Autodesk Inventor part; units mm, degrees
ref_plane "YZ Plane" through (0, 0, 0) normal (1, 0, 0) x (0, 1, 0)
ref_plane "XZ Plane" through (0, 0, 0) normal (0, 1, 0) x (-1, 0, 0)
ref_plane "XY Plane" through (0, 0, 0) normal (0, 0, 1) x (1, 0, 0)
sketch "Sketch1" plane through (0, 0, 0) normal (0, 0, 1) x (1, 0, 0)
  line L0 (0, 2.4078) -> (0, -18.8352)
  line L1 (-12.7, 4.1621) -> (-12.7, -19.6361)
  line L2 (-20.3324, 0) -> (-11.9249, 0)
  circle A0 centre (-12.7, 12.7) radius 3.175
  circle A1 centre (-12.7, -12.7) radius 3.175
  line L3 (-26.1938, 25.4) -> (-0.7938, 25.4)
  line L4 (-0.7938, 25.4) -> (-0.7937, -25.4)
  line L5 (-0.7937, -25.4) -> (-26.1937, -25.4)
  line L6 (-26.1937, -25.4) -> (-26.1938, 25.4)
  point P0 (0, 0)
  dimension "d0" = 12.7
  dimension "d1" = 25.4
  dimension "d2" = 25.4
  dimension "d3" = 6.35
  dimension "d4" = 6.35
  dimension "d5" = 1.5875
  dimension "d6" = 25.4
  dimension "d7" = 50.8
  dimension "d8" = 12.7
extrude "Extrusion1" add sketch "Sketch1" along normal blind 6.35
sketch "Sketch2" plane through (0, 0, 6.35) normal (0, 0, 1) x (1, 0, 0)
  line L0 (-0.7938, 25.4) -> (-26.1938, 25.4)
  line L1 (-0.7937, -25.4) -> (-0.7938, 25.4)
  line L2 (-5.8738, 25.4) -> (-0.7937, 25.4)
  line L3 (-0.7937, 25.4) -> (-0.7937, -25.4)
  line L4 (-0.7937, -25.4) -> (-5.8737, -25.4)
  line L5 (-5.8737, -25.4) -> (-5.8738, 25.4)
  point P0 (0, 0)
  dimension "d11" = 5.08
extrude "Extrusion2" add sketch "Sketch2" along normal blind 12.7
properties part number "diffuser holder"
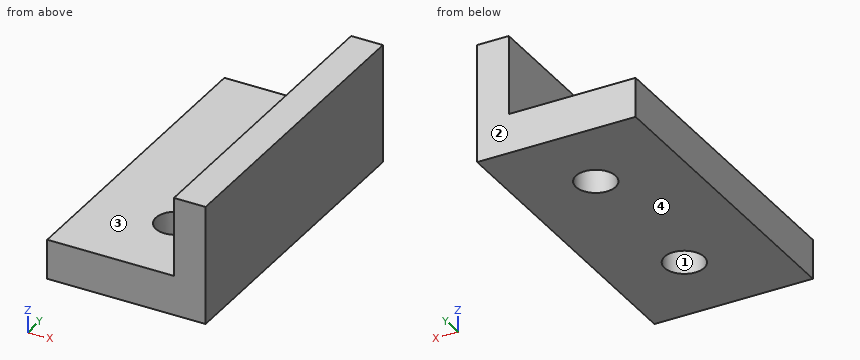
Here's how the part is built. I have some questions about the finished solid (model axes, mm). Face numbers are marked on the shaded views. A direction names the side the tool comes from. Round coordinates to 2 decimals unless told otherwise and drop trailing zeros. Write each loop counter-clockwise with the first axis right and the second up, starting at its lowest first coordinate (ties: lowest second). Pieces come first, ordered by that corner, then holes.
1. Suppose I cut it at A-A (x = -12.7). List the corners of the cut face in (y, z) for me (3 decimals), and give its area (3 significant figures).
2. Will these pins go through, and if not, where does the flat tip stop? pin 1 Ø12 at (x, y) = (-14, -10) entering from +Z; pin 2 Ø10 at (x, y) = (-20.5, -11) entering from -Z; pin 3 Ø6.5 at (y, z) = (-12.5, 15.5) entering from -X; pin 4 Ø5 at (x, y) = (-12.7, -12.7) entering from -Z.
3. I need wall thicknesses on L1, parallel to Y at x = -12.7, z = 5.25 (3 decimals); L2, parallel to Y at x = -14.5, z = 3.5; L3, parallel to Z at x = -24.5, y = -7. Which ranges of each line are inside material? Lowest first, please.
4. Suppose I cut it at D-D (z = 10.75). List the corners of the cut face in (x, y) for me.
5. Suppose I cut it at B-B (y = 12.7). List the corners of the cut face in (x, z) for me (3 decimals).
6. If we mould it in two halves opening along X, with no side actions, what happens to the marked faces 1 and 2? For each: released by +X, released by -X, zero draft, split by the parting line, or undercut.
7. Suppose I cut it at C-C (z = 5). List the corners of the cut face in (x, y) for me (3 decimals), and give its area (3 significant figures).
8. For the marked faces 3 and 4, which set-ups out of +Z, -Z, +X, -X, +Y, -Y let a thin tool reach every point of the face, with its end or its side?
Answer sheet:
1. outline: (-25.4, 0) - (-15.875, 0) - (-15.875, 6.35) - (-25.4, 6.35) - close; (-9.525, 0) - (9.525, 0) - (9.525, 6.35) - (-9.525, 6.35) - close; (15.875, 0) - (25.4, 0) - (25.4, 6.35) - (15.875, 6.35) - close
1. area: 242 mm2
2. pin 1: stops at z = 6.35
2. pin 2: stops at z = 0
2. pin 3: stops at x = -5.87
2. pin 4: passes through
3. L1: y = -25.4 to -15.875, -9.525 to 9.525, 15.875 to 25.4
3. L2: y = -25.4 to -15.32, -10.08 to 10.08, 15.32 to 25.4
3. L3: z = 0 to 6.35
4. outline: (-5.87, -25.4) - (-0.79, -25.4) - (-0.79, 25.4) - (-5.87, 25.4) - close
5. outline: (-26.194, 0) - (-15.875, 0) - (-15.875, 6.35) - (-26.194, 6.35) - close; (-9.525, 0) - (-0.794, 0) - (-0.794, 19.05) - (-5.874, 19.05) - (-5.874, 6.35) - (-9.525, 6.35) - close
6. face 1: undercut
6. face 2: zero draft
7. outline: (-26.194, -25.4) - (-0.794, -25.4) - (-0.794, 25.4) - (-26.194, 25.4) - close; hole circle Ø6.35 at (-12.7, -12.7); hole circle Ø6.35 at (-12.7, 12.7)
7. area: 1,230 mm2
8. face 3: +Z, -X, +Y, -Y
8. face 4: -Z, +X, -X, +Y, -Y
